Could you check a few things on this model? Use its own coordinates, in mm. Face numbers are marked on the shaded views. Give positions to 0.01 mm unless a question says otherwise; leave off trailing zeros. Order: outer loops, then holes, each group sorted by start corner. A loop starts at its lowest first (then second) coordinate and runs counter-clockwise, first axis right, second up. Notation, with made-up numbers: M 48.5,51 L 99.5,51 A26 ccw 99.5,73 Z; hole C 9,29 d3. An arc over 180 degrees is marked long. Return JSON: item names as keys, results as strings. Group by question number.
```python
from build123d import *

# Parameters (mm, degrees)
F1_DEPTH  = 15
F2_R      = 1.25
F3_DEPTH  = 25
F4_T      = 4
F5_R      = 1.25
F6_DEPTH  = 25
F7_W      = 56
F7_H      = 4
F8_DEPTH  = 25
F9_W      = 25
F9_H      = 6
F10_DEPTH = 11
F11_R     = 1
F13_D     = 2.5
F13_DEPTH = 10
F13_TIP   = 0.7510757738
F15_D     = 2.5
F15_DEPTH = 10
F15_TIP   = 0.7510757738
F16_R     = 1.25
F17_DEPTH = 11
F18_R     = 1
F20_D     = 2.5
F20_DEPTH = 10
F20_TIP   = 0.7510757738
F21_W     = 6
F21_H     = 56
F22_DEPTH = 25
F24_D     = 5
F24_DEPTH = 100
F24_TIP   = 1.5021515476
F25_R     = 1.25
F26_DEPTH = 5


# Not quite as in the source:
# - a shell that OpenCascade refuses in one call is made with other operations: the cavity is built on its own and cut out


with BuildPart() as f1:
    # F0 (on Front) → F1 (new body)
    with BuildSketch(Plane.XZ):
        with BuildLine():
            Line((-75, -60), (75, -60))
            ThreePointArc((75, -60), (78.5355339059, -58.5355339059), (80, -55))
            Line((80, -55), (80, 55))
            ThreePointArc((80, 55), (78.5355339059, 58.5355339059), (75, 60))
            Line((75, 60), (-75, 60))
            ThreePointArc((-75, 60), (-78.5355339059, 58.5355339059), (-80, 55))
            Line((-80, 55), (-80, -55))
            ThreePointArc((-80, -55), (-78.5355339059, -58.5355339059), (-75, -60))
        make_face()
    extrude(amount=F1_DEPTH)

    # F2 (on Front) → F3 (cut)
    with BuildSketch(Plane.XZ):
        with Locations((-75, 55)):
            Circle(F2_R)
        with Locations((75, 55)):
            Circle(F2_R)
        with Locations((75, -55)):
            Circle(F2_R)
        with Locations((-75, -55)):
            Circle(F2_R)
    extrude(amount=F3_DEPTH, mode=Mode.SUBTRACT)

    # F4: shell of thickness 4, made by hand


with BuildPart() as f4_core1:
    # F4_t2: copy of F1
    add(f1.part)

    # the walls: a layer under each face that stays
    f4_faces = [f4_core1.faces().sort_by_distance(p)[0] for p in [
        (0, -7.5, -60),
        (-78.5355339059, -7.5, -58.5355339059),
        (78.5355339059, -7.5, -58.5355339059),
        (0, 0, 0),
        (-80, -7.5, 0),
        (80, -7.5, 0),
        (-78.5355339059, -7.5, 58.5355339059),
        (78.5355339059, -7.5, 58.5355339059),
        (0, -7.5, 60),
        (-76.25, -7.5, -55),
        (73.75, -7.5, -55),
        (-76.25, -7.5, 55),
        (73.75, -7.5, 55),
    ]]
    thicken(f4_faces, amount=-F4_T, mode=Mode.SUBTRACT)


with BuildPart() as f1_1:
    add(f1.part)

    # what is left inside the walls is the cavity
    f4_cavity = [f4_core1.part.solids().sort_by_distance(p)[0] for p in [
        (0, -4.04, -18.666667),
    ]]
    add(f4_cavity, mode=Mode.SUBTRACT)

    # F5 (on face) → F6 (cut)
    with BuildSketch(Plane.XZ.offset(4)):
        with Locations((3.5, 34.4)):
            Circle(F5_R)
        with Locations((52.5, 34.4)):
            Circle(F5_R)
        with Locations((52.5, -23.6)):
            Circle(F5_R)
        with Locations((3.5, -23.6)):
            Circle(F5_R)
    extrude(amount=-F6_DEPTH, mode=Mode.SUBTRACT)

    # F7 (on face) → F8 (cut)
    with BuildSketch(Plane.XZ.offset(4)):
        with Locations((26.75, 58)):
            Rectangle(F7_W, F7_H)
    extrude(amount=F8_DEPTH, mode=Mode.SUBTRACT)

    # F9 (on face) → F10 (join)
    with BuildSketch(Plane.XZ.offset(4)):
        with Locations((-47.5, 53)):
            Rectangle(F9_W, F9_H)
    extrude(amount=F10_DEPTH)

    # F11
    f11_edges = [f1_1.edges().sort_by_distance(p)[0] for p in [
        (-60, -9.5, 56),
        (-60, -9.5, 50),
        (-35, -9.5, 50),
        (-35, -9.5, 56),
    ]]
    fillet(f11_edges, radius=F11_R)

    # F13
    with Locations(Plane.XZ.offset(15)):
        with Locations((-56, 56), (-39, 56)):
            Hole(F13_D / 2, depth=F13_DEPTH)
            with Locations((0, 0, -(F13_DEPTH + F13_TIP / 2))):  # 118° drill point
                Cone(0, F13_D / 2, F13_TIP, mode=Mode.SUBTRACT)

    # F15
    with Locations(Plane.XZ.offset(4)):
        with Locations((-49, 45), (-73, 45), (-73, 21), (-49, 21)):
            Hole(F15_D / 2, depth=F15_DEPTH)
            with Locations((0, 0, -(F15_DEPTH + F15_TIP / 2))):  # 118° drill point
                Cone(0, F15_D / 2, F15_TIP, mode=Mode.SUBTRACT)

    # F16 (on face) → F17 (join)
    with BuildSketch(Plane.XZ.offset(4)):
        with BuildLine():
            Line((-76, 14), (-76, 4))
            Line((-76, 4), (-46, 4))
            ThreePointArc((-46, 4), (-45.2928932188, 4.2928932188), (-45, 5))
            Line((-45, 5), (-45, 13))
            ThreePointArc((-45, 13), (-45.2928932188, 13.7071067812), (-46, 14))
            Line((-46, 14), (-76, 14))
        make_face()
        with Locations((-70, 9)):
            Circle(F16_R, mode=Mode.SUBTRACT)
    extrude(amount=F17_DEPTH)

    # F18
    f18_edges = [f1_1.edges().sort_by_distance(p)[0] for p in [
        (-76, -9.5, 14),
        (-76, -9.5, 4),
        (-69.846118, -9.5, 56),
        (-76, -9.5, 49.846118),
        (-76, -9.5, -49.846118),
        (-69.846118, -9.5, -56),
        (69.846118, -9.5, -56),
        (76, -9.5, -49.846118),
        (76, -9.5, 49.846118),
        (69.846118, -9.5, 56),
    ]]
    fillet(f18_edges, radius=F18_R)

    # F20
    with Locations(Plane.XZ.offset(4)):
        with Locations((-61.220435021, 43.0927334726), (-61.220435021, 38.0927334726), (-68.2273637709, 40.2273637709), (-71.220435021, 33.0927334726), (-66.220435021, 33.0927334726), (-68.1331846448, 25.8668153552), (-61.220435021, 28.0927334726), (-61.220435021, 23.0927334726), (-53.9945169036, 40.0054830964), (-56.220435021, 33.0927334726), (-54.0858047227, 26.0858047227), (-51.220435021, 33.0927334726)):
            Hole(F20_D / 2, depth=F20_DEPTH)
            with Locations((0, 0, -(F20_DEPTH + F20_TIP / 2))):  # 118° drill point
                Cone(0, F20_D / 2, F20_TIP, mode=Mode.SUBTRACT)

    # F21 (on face) → F22 (cut)
    with BuildSketch(Plane.XZ.offset(4)):
        with Locations((-6, 5.4)):
            Rectangle(F21_W, F21_H)
    extrude(amount=-F22_DEPTH, mode=Mode.SUBTRACT)

    # F24 (one way)
    with BuildSketch(Plane(origin=(0, 0, 0), x_dir=(0, 1, 0), z_dir=(-1, 0, 0))):
        with Locations((-9.5, 35), (-9.5, 45)):
            Circle(F24_D / 2)
    extrude(amount=-F24_DEPTH, mode=Mode.SUBTRACT)
    with Locations(Plane(origin=(0, 0, 0), x_dir=(0, 1, 0), z_dir=(-1, 0, 0))):
        with Locations((-9.5, 35), (-9.5, 45)):
            with Locations((0, 0, -(F24_DEPTH + F24_TIP / 2))):  # 118° drill point
                Cone(0, F24_D / 2, F24_TIP, mode=Mode.SUBTRACT)

    # F25 (on face) → F26 (cut)
    with BuildSketch(Plane.XZ.offset(4)):
        with Locations((-28, 45)):
            Circle(F25_R)
        with Locations((-28, 8)):
            Circle(F25_R)
    extrude(amount=-F26_DEPTH, mode=Mode.SUBTRACT)


solid = f1_1.part
```
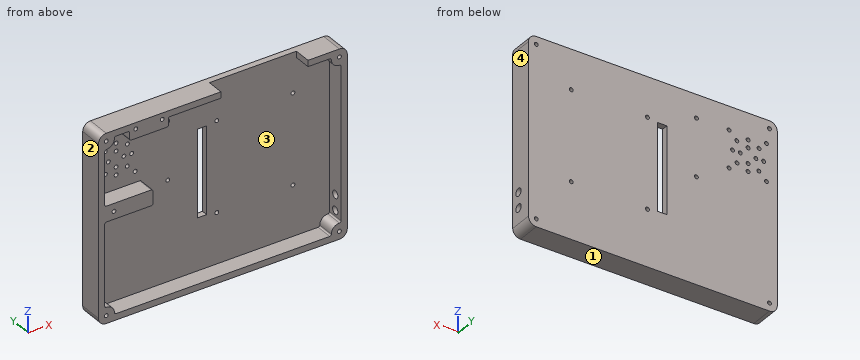
1. If we mould it in two halves opening along X, with no side actions, what happens to the marked faces 1, 2, 3 and 4? For each: pulls with the +X half, pulls with the -X half, needs draft (parallel to the pull), parting line crosses it, or undercut.
2. For pin 1 (4 mm diameter, centred on x = -38.5, z = 41.5, fed in from -Y); pin 2 (4 mm diameter, centred on x = -73, z = 21, fed in from +Y), each with a flat end and sliding along its axis, tell me the tip position at first contact or that it passes through.
3. I need wall thicknesses on L1, parallel to Z at x = 3.5, y = -1.35; L2, parallel to X at y = -5, z = 3; L3, parallel to Y at x = 78.7, z = -35. Which ranges of each line are inside material? Lowest first, please. Write a range as from..to.
4. Imagine slicing it at C-C, the plane x = 45.5. Please give me the cut outline in (y, z).
5. Imagine slicing it at B-B, the plane z = -35. Please give me the cut outline in (x, y).
6. Imagine slicing it at A-A, the plane z = -16.5. Please give me the cut outline in (x, y).
Values:
{
 "1": {"face 1": "needs draft", "face 2": "pulls with the -X half", "face 3": "undercut", "face 4": "pulls with the +X half"},
 "2": {"pin 1": "stops at y = -4", "pin 2": "stops at y = 0"},
 "3": {"L1": "z = -60..-24.85, -22.35..33.15, 35.65..60", "L2": "x = -80..-76, 76..80", "L3": "y = -15..-12, -7..0"},
 "4": {"outline": "M -15,-60 L 0,-60 L 0,60 L -4,60 L -4,-56 L -15,-56 Z"},
 "5": {"outline": "M -80,-15 L -76,-15 L -76,-4 L 76,-4 L 76,-7 L 80,-7 L 80,0 L -80,0 Z; M 76,-15 L 80,-15 L 80,-12 L 76,-12 Z"},
 "6": {"outline": "M -80,-15 L -76,-15 L -76,-4 L -9,-4 L -9,0 L -80,0 Z; M -3,-4 L 76,-4 L 76,-15 L 80,-15 L 80,0 L -3,0 Z"}
}
